```python
from build123d import *

# Parameters (mm, degrees)
EXTRUDE_1_DEPTH     = 1.6
EXTRUDE_2_DEPTH     = 0.5
SKETCH_3_W          = 0.4
SKETCH_3_H          = 1.6
SKETCH_3_W_2        = 0.6
SKETCH_3_H_2        = 0.4
SKETCH_3_H_3        = 0.6
CUT_EXTRUDE_1_DEPTH = 0.5


with BuildPart() as part:
    # 草图1 → 凸台-拉伸1 (new body)
    with BuildSketch(Plane(origin=(0, 0, 0), x_dir=(1, 0, 0), z_dir=(0, 1, 0))):
        with BuildLine():
            Line((-8.8, 1.15), (8.8, 1.15))
            ThreePointArc((8.8, 1.15), (9.95, 0), (8.8, -1.15))
            Line((8.8, -1.15), (-8.8, -1.15))
            ThreePointArc((-8.8, -1.15), (-9.95, 0), (-8.8, 1.15))
        make_face()
    extrude(amount=EXTRUDE_1_DEPTH)

    # 草图2 → 凸台-拉伸2 (add)
    with BuildSketch(Plane.XZ):
        with BuildLine():
            Line((-8.8, -2.15), (8.8, -2.15))
            ThreePointArc((8.8, -2.15), (10.95, 0), (8.8, 2.15))
            Line((8.8, 2.15), (-8.8, 2.15))
            ThreePointArc((-8.8, 2.15), (-10.95, 0), (-8.8, -2.15))
        make_face()
    extrude(amount=EXTRUDE_2_DEPTH)

    # 草图3 → 切除-拉伸1 (cut)
    with BuildSketch(Plane(origin=(0, 1.6, 0), x_dir=(1, 0, 0), z_dir=(0, 1, 0))):
        with Locations((8, 0)):
            Rectangle(SKETCH_3_W, SKETCH_3_H)
        with Locations((-8.5, 0)):
            Rectangle(SKETCH_3_W_2, SKETCH_3_H_2)
        with Locations((-8, 0)):
            Rectangle(SKETCH_3_W, SKETCH_3_H_2)
        with Locations((-8, 0.5)):
            Rectangle(SKETCH_3_W, SKETCH_3_H_3)
        with Locations((-7.5, 0)):
            Rectangle(SKETCH_3_W_2, SKETCH_3_H_2)
        with Locations((-8, -0.5)):
            Rectangle(SKETCH_3_W, SKETCH_3_H_3)
    extrude(amount=-CUT_EXTRUDE_1_DEPTH, mode=Mode.SUBTRACT)


solid = part.part
```
CAD build for the part. Positions are in the model's coordinates, mm. A direction names the side the tool comes from. Round coordinates to 2 decimals unless told otherwise and drop trailing zeros. Write each loop counter-clockwise with the first axis right and the second up, starting at its lowest first coordinate (ties: lowest second). Pieces come first, ordered by that corner, then holes. Notation, with made-up numbers: (0, -38.75) -> (55, -38.75) arc R16 ccw to (55, -32.75) -> close; hole circle Ø2 at (23, -19.75). An arc over 180 degrees is marked (long way). Answer in a Markdown table with one row per item. Add a question column.
Item 1: Drill centre lines: line 1 (Z direction, x = 8, y = 0.35); line 2 (Y direction, x = 2.5, z = 1.45); line 3 (X direction, y = 0.55, z = 0.7). Where is each one in solid material? Low to high. Write a range as from..to.
Item 2: Drop flat-ended pins along their axis: pin 1 Ø0.6 at (y, z) = (1.5, 0.5) entering from +X; pin 2 Ø0.6 at (x, y) = (-7.5, 1.5) entering from -Z. Give the stop position or say it passes through.
Item 3: Saw through at A-A, the plane y = 1.35. Write the cut outline in (x, z).
Item 4: Mould opens along X. For faces 1 (the face through (-10.95, -0.25, 0.05)), 2 (the face through (-8, 1.1, 0)), 3 (the face through (10.95, -0.25, -0.05)) say: pulls with the +X half, pulls with the -X half, needs draft (parallel to the pull), parting line crosses it, or undercut.
Item 5: Which spindle directions (+Z, -Z, +X, -X, +Y, -Y) get a long thin tool onto all of the face, cutting with end or side? Do faces 4 (the face through (0, 1, -1.15)), 5 (the face through (0, 1, 1.15)), 6 (the face through (9.95, 0.79, -0.03)), 7 (the face through (-9.95, 0.79, 0.03)), 8 (the face through (0, -0.5, 0)). Say none if no direction does.
Item 6: Saw through at D-D, the plane y = -0.2. Write the cut outline in (x, z).
Item 7: Saw through at B-B, the plane z = 0. Write the cut outline in (x, y), then the cut area to 3 significant figures.
Item 8: Saw through at C-C, the plane x = -0.5. Write the cut outline in (y, z).
Findings below:
| question | item | result |
|---|---|---|
| 1 | line 1 | z = -1.15..1.15 |
| 1 | line 2 | y = -0.5..0 |
| 1 | line 3 | x = -9.71..9.71 |
| 2 | pin 1 | stops at x = 9.93 |
| 2 | pin 2 | stops at z = -1.15 |
| 3 | outline | (-8.8, -1.15) -> (8.8, -1.15) arc R1.15 ccw to (8.8, 1.15) -> (-8.8, 1.15) arc R1.15 ccw to start; hole (-8.8, -0.2) -> (-8.2, -0.2) -> (-8.2, -0.8) -> (-7.8, -0.8) -> (-7.8, -0.2) -> (-7.2, -0.2) -> (-7.2, 0.2) -> (-7.8, 0.2) -> (-7.8, 0.8) -> (-8.2, 0.8) -> (-8.2, 0.2) -> (-8.8, 0.2) -> close; hole (7.8, -0.8) -> (8.2, -0.8) -> (8.2, 0.8) -> (7.8, 0.8) -> close |
| 4 | face 1 | pulls with the -X half |
| 4 | face 2 | undercut |
| 4 | face 3 | pulls with the +X half |
| 5 | face 4 | -Z, +X, -X, +Y |
| 5 | face 5 | +Z, +X, -X, +Y |
| 5 | face 6 | +X, +Y |
| 5 | face 7 | -X, +Y |
| 5 | face 8 | +Z, -Z, +X, -X, -Y |
| 6 | outline | (-8.8, -2.15) -> (8.8, -2.15) arc R2.15 ccw to (8.8, 2.15) -> (-8.8, 2.15) arc R2.15 ccw to start |
| 7 | outline | (-10.95, -0.5) -> (10.95, -0.5) -> (10.95, 0) -> (9.95, 0) -> (9.95, 1.6) -> (8.2, 1.6) -> (8.2, 1.1) -> (7.8, 1.1) -> (7.8, 1.6) -> (-7.2, 1.6) -> (-7.2, 1.1) -> (-8.8, 1.1) -> (-8.8, 1.6) -> (-9.95, 1.6) -> (-9.95, 0) -> (-10.95, 0) -> close |
| 7 | area | 41.8 mm^2 |
| 8 | outline | (-0.5, -2.15) -> (0, -2.15) -> (0, -1.15) -> (1.6, -1.15) -> (1.6, 1.15) -> (0, 1.15) -> (0, 2.15) -> (-0.5, 2.15) -> close |
